Here's the drawing with two shaded views (mm, measured from the low corner). I have some questions. Coordinates: 2 decimals unless noted, no trailing zeros. Write each loop counter-clockwise with the first axis right and the second up, starting at its lowest first coordinate (ties: lowest second). Pieces come first, ordered by that corner, then holes. Notation, with made-up numbers: (-10.75, -23.75) -> (30.25, -23.75) arc R20 cw to (30.25, 9.25) -> close; hole circle Ø11 at (83.25, 68.5). An arc over 180 degrees is marked (long way). Answer in a Markdown table with one row per item. Add a question column.
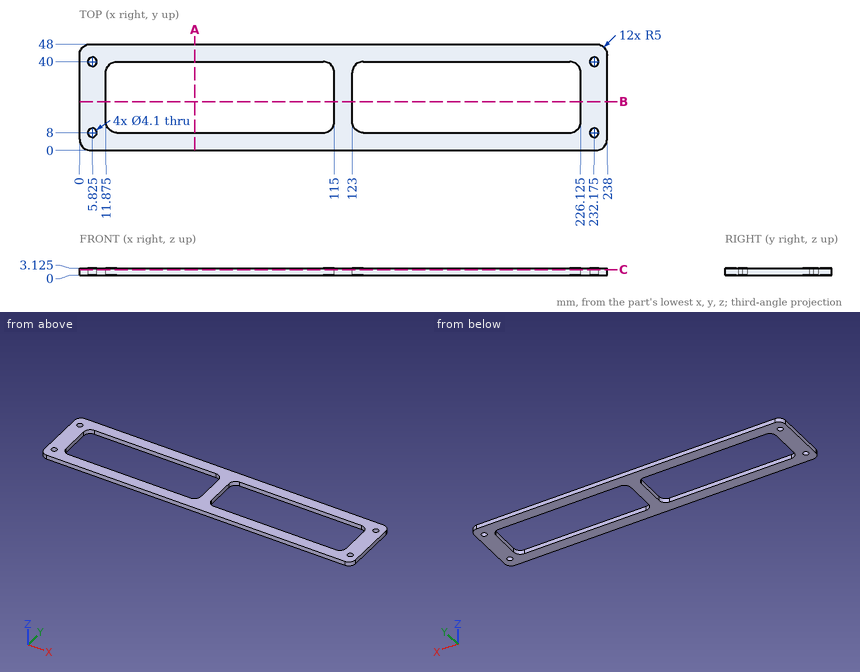
Q1. Imagine slicing it at B-B on y = 22. Please give me the cut outline in (x, z) (3 decimals), plus the area to 3 significant figures.
Q2. I need wall thicknesses on line 1 (X direction, y = 14, z = 2.4) (3 decimals); line 2 (Y direction, x = 196, z = 2.6); line 3 (Y direction, x = 114, z = 0.85). Which ranges of each line are inside material? Lowest first, please. Write a range as [from, to].
Q3. Imagine slicing it at A-A on x = 52. Please give me the cut outline in (y, z) (3 decimals).
Q4. I'm going to push a flat-ended pin straight in: P1, Ø1.6, axis at x = 64.5, z = 1, coming from the -Y side. Where does the tip first touch, or does it pass through?
Q5. Imagine slicing it at C-C on z = 2.55. Please give me the cut outline in (x, y) (3 decimals), plus the area to 3 significant figures.
Result sheet:
| question | item | result |
|---|---|---|
| 1 | outline | (0, 0) -> (11.875, 0) -> (11.875, 3.125) -> (0, 3.125) -> close; (115, 0) -> (123, 0) -> (123, 3.125) -> (115, 3.125) -> close; (226.125, 0) -> (238, 0) -> (238, 3.125) -> (226.125, 3.125) -> close |
| 1 | area | 99.2 mm^2 |
| 2 | line 1 | x = [0, 11.875], [115, 123], [226.125, 238] |
| 2 | line 2 | y = [0, 8], [40, 48] |
| 2 | line 3 | y = [0, 10], [38, 48] |
| 3 | outline | (0, 0) -> (8, 0) -> (8, 3.125) -> (0, 3.125) -> close; (40, 0) -> (48, 0) -> (48, 3.125) -> (40, 3.125) -> close |
| 4 | P1 | stops at y = 0 |
| 5 | outline | (0, 5) arc R5 ccw to (5, 0) -> (233, 0) arc R5 ccw to (238, 5) -> (238, 43) arc R5 ccw to (233, 48) -> (5, 48) arc R5 ccw to (0, 43) -> close; hole circle Ø4.1 at (5.825, 8); hole circle Ø4.1 at (5.825, 40); hole (11.875, 13) arc R5 ccw to (16.875, 8) -> (110, 8) arc R5 ccw to (115, 13) -> (115, 35) arc R5 ccw to (110, 40) -> (16.875, 40) arc R5 ccw to (11.875, 35) -> close; hole (123, 13) arc R5 ccw to (128, 8) -> (221.125, 8) arc R5 ccw to (226.125, 13) -> (226.125, 35) arc R5 ccw to (221.125, 40) -> (128, 40) arc R5 ccw to (123, 35) -> close; hole circle Ø4.1 at (232.175, 8); hole circle Ø4.1 at (232.175, 40) |
| 5 | area | 4,790 mm^2 |
